Input: part model. Units: mm. Frame: model coordinates. Face numbers are marked on the shaded views. A direction names the side the tool comes from. Give positions to 0.01 mm unless a question says otherwise; leave off trailing zeros. Loops run counter-clockwise (first coordinate to the right, second up) from the corner with the lowest first, then second, coordinate; pieces in that order, holes last.
from build123d import *

# Parameters (mm, degrees)
SKETCH_R        = 1.55
PAD_DEPTH       = 6.3
SKETCH002_W     = 5.6
SKETCH002_H     = 5.6
POCKET_DEPTH    = 2
PAD001_DEPTH    = 7.7
SKETCH003_R     = 1.65
POCKET001_DEPTH = 6.901
SKETCH004_W     = 5.6
SKETCH004_H     = 5.6
POCKET002_DEPTH = 2
SKETCH005_W     = 10
SKETCH005_H     = 7
PAD002_DEPTH    = 11.9
SKETCH006_R     = 1.6
PAD003_DEPTH    = 7.5
PAD004_DEPTH    = 11.9
FILLET_R        = 5
CHAMFER_SIZE    = 7


with BuildPart() as part:
    # Sketch → Pad (new body)
    with BuildSketch(Plane.YZ):
        Polygon((-6.9, -4.5), (0, -4.5), (0, -19), (-15, -19), (-15, -11), (-6.9, -11), align=None)
        with Locations((-11, -15)):
            Circle(SKETCH_R, mode=Mode.SUBTRACT)
        with Locations((-4, -15)):
            Circle(SKETCH_R, mode=Mode.SUBTRACT)
    extrude(amount=PAD_DEPTH)

    # Sketch002 (on Face9 of Pad) → Pocket (cut)
    with BuildSketch(Plane(origin=(0, 0, 0), x_dir=(0, 1, 0), z_dir=(-1, 0, 0))):
        with Locations((-4, 15)):
            Rectangle(SKETCH002_W, SKETCH002_H)
        with Locations((-11, 15)):
            Rectangle(SKETCH002_W, SKETCH002_H)
    extrude(amount=-POCKET_DEPTH, mode=Mode.SUBTRACT)

    # Sketch001 (on Face1 of Pad) → Pad001 (join)
    with BuildSketch(Plane(origin=(0, 0, -4.5), x_dir=(0, -1, 0), z_dir=(0, 0, 1))):
        Polygon((0, 0), (0, -16), (10, -16), (10, -9), (6.9, -9), (6.9, -2.7), (10, -2.7), (10, 0), align=None)
    extrude(amount=-PAD001_DEPTH)

    # Sketch003 (on Face1 of Pad001) → Pocket001 (cut, through all)
    with BuildSketch(Plane(origin=(0, -6.9, 0), x_dir=(0, 0, -1), z_dir=(0, -1, 0))):
        with Locations((8.15, -5.85)):
            Circle(SKETCH003_R)
        with Locations((8.15, 3.15)):
            Circle(SKETCH003_R)
    extrude(amount=-POCKET001_DEPTH, mode=Mode.SUBTRACT)

    # Sketch004 (on Face10 of Pocket001) → Pocket002 (cut)
    with BuildSketch(Plane.ZX):
        with Locations((-8.15, 3.15)):
            Rectangle(SKETCH004_W, SKETCH004_H)
        with Locations((-8.15, -5.85)):
            Rectangle(SKETCH004_W, SKETCH004_H)
    extrude(amount=-POCKET002_DEPTH, mode=Mode.SUBTRACT)

    # Sketch005 (on Face5 of Pocket002) → Pad002 (join)
    with BuildSketch(Plane(origin=(0, 0, -4.5), x_dir=(0, -1, 0), z_dir=(0, 0, 1))):
        with Locations((5, -12.5)):
            Rectangle(SKETCH005_W, SKETCH005_H)
    extrude(amount=PAD002_DEPTH)

    # Sketch006 (on Face35 of Pad002) → Pad003 (join)
    with BuildSketch(Plane(origin=(0, -10, 0), x_dir=(0, 0, -1), z_dir=(0, -1, 0))):
        with Locations((-2.05, -12.7)):
            Circle(SKETCH006_R)
        with Locations((2.05, -12.7)):
            Circle(SKETCH006_R)
    extrude(amount=PAD003_DEPTH)

    # Sketch007 (on Face7 of Pad003) → Pad004 (join)
    with BuildSketch(Plane(origin=(0, 0, -4.5), x_dir=(0, -1, 0), z_dir=(0, 0, 1))):
        with BuildLine():
            Line((10, -2.5), (1.15, -2.5))
            ThreePointArc((1.15, -0.2), (0, -1.35), (1.15, -2.5))
            Line((1.15, -0.2), (10, -0.2))
            Line((10, -0.2), (10, -2.5))
        make_face()
    extrude(amount=PAD004_DEPTH)

    # Fillet
    fillet_edges = [part.edges().sort_by_distance(p)[0] for p in [
        (-16, -5, 7.4),
    ]]
    fillet(fillet_edges, radius=FILLET_R)

    # Chamfer
    chamfer_edges = [part.edges().sort_by_distance(p)[0] for p in [
        (-16, -5, -12.2),
    ]]
    chamfer(chamfer_edges, length=CHAMFER_SIZE)


solid = part.part
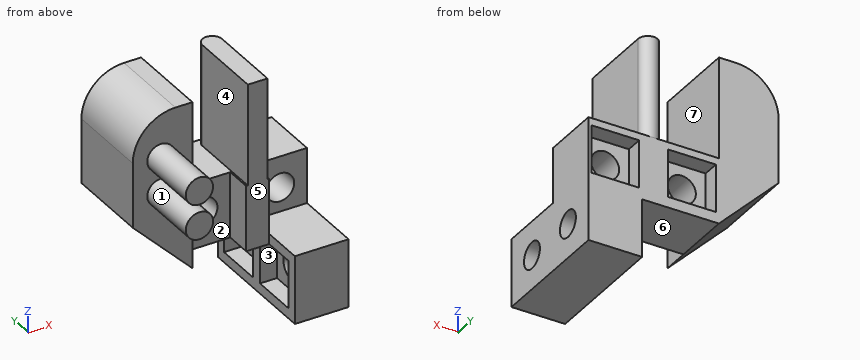
(1) Reachability of the marked faces 1, 2, 3 and 4 from +Z, -Z, +X, -X, +Y, -Y: full face, straight path, thin tool, end or side. Return the list, or none.
Values follow:
face 1: -Y
face 2: +Z, -Z, -Y
face 3: -X
face 4: +Z, +Y, -Y
(2) Ray query, probe 1 along Y at (x, z) = (1.25, -12.5); probe 2 along Y at (x, z) = (3.5, -15); probe 3 along X at (y, z) = (-4.7, -8.15). Return the intervals inside material, ascending.
Values follow:
probe 1: y = -15 to -13.8, -8.2 to -6.8, -1.2 to 0
probe 2: y = -15 to -12.55, -9.45 to -5.55, -2.45 to 0
probe 3: x = -13.05 to -7.5, -4.2 to 1.5, 4.8 to 6.3
(3) Cut plane D-D (y = -7.5). Return the cut outline in (x, z).
Values follow:
outline: (-16, -5.2) - (-9, -12.2) - (-9, 7.4) - (-11, 7.4) arc R5 ccw to (-16, 2.4) - close; (-2.7, -12.2) - (0, -12.2) - (0, -19) - (6.3, -19) - (6.3, -11) - (0, -11) - (0, -4.5) - (-0.2, -4.5) - (-0.2, 7.4) - (-2.5, 7.4) - (-2.5, -4.5) - (-2.7, -4.5) - close
(4) Cut plane B-B (z = -2.05). Return the cut outline in (x, y), and give its area (3 significant figures).
Values follow:
outline: (-16, -10) - (-14.3, -10) - (-14.3, -17.5) - (-11.1, -17.5) - (-11.1, -10) - (-9, -10) - (-9, 0) - (-16, 0) - close; (-2.5, -10) - (-0.2, -10) - (-0.2, -1.15) arc R1.15 ccw to (-2.5, -1.15) - close
area: 116 mm2
(5) Mould query, pull axis Y, two halves, no side actions, for the marked faces 5, 6 and 7. Classes: +Y half, -Y half, draft (parallel to the pull), parting line (faces both ways), or undercut.
Values follow:
face 5: -Y half
face 6: undercut
face 7: draft
(6) Cut plane A-A (x = 3.15). Return the cut outline in (y, z), and give its area (3 significant figures).
Values follow:
outline: (-15, -19) - (0, -19) - (0, -10.95) - (-2, -10.95) - (-2, -9.8) - (-6.9, -9.8) - (-6.9, -11) - (-15, -11) - close; (-6.9, -6.5) - (-2, -6.5) - (-2, -5.35) - (0, -5.35) - (0, -4.5) - (-6.9, -4.5) - close; hole circle Ø3.1 at (-11, -15); hole circle Ø3.1 at (-4, -15)
area: 122 mm2
(7) Cut plane C-C (y = -11). Return the cut outline in (x, z), and give its area (3 significant figures).
Values follow:
outline: circle Ø3.2 at (-12.7, -2.05); circle Ø3.2 at (-12.7, 2.05); (0, -19) - (6.3, -19) - (6.3, -16.55) - (2, -16.55) - (2, -17.8) - (0, -17.8) - close; (0, -12.2) - (2, -12.2) - (2, -13.45) - (6.3, -13.45) - (6.3, -11) - (0, -11) - close
area: 42.0 mm2
(8) Pin query (flat end, axial travel): pin 1 Ø6 at (x, z) = (-11, -12) entering from -Y; pin 2 Ø2.5 at (y, z) = (-5.5, 2) entering from +X; pin 3 Ø1.5 at (y, z) = (-8, -7.5) entering from +X; pin 4 Ø2.5 at (x, z) = (3.15, -8.15) entering from -Y. Return the tip coordinate at first contact, or that it passes through.
Values follow:
pin 1: stops at y = -10
pin 2: stops at x = -0.2
pin 3: stops at x = 0
pin 4: passes through
